Autodesk Inventor part; units mm, degrees
ref_plane "YZ Plane" through (0, 0, 0) normal (1, 0, 0) x (0, 1, 0)
ref_plane "XZ Plane" through (0, 0, 0) normal (0, 1, 0) x (-1, 0, 0)
ref_plane "XY Plane" through (0, 0, 0) normal (0, 0, 1) x (1, 0, 0)
sketch "Sketch1" plane through (0, 0, 0) normal (0, 0, 1) x (1, 0, 0)
  circle A0 centre (0, 0) radius 1.725
  dimension "d0" = 3.45
extrude "Extrusion1" add sketch "Sketch1" along normal blind 0.5
sketch "Sketch2" plane through (0, 0, 0.5) normal (0, 0, 1) x (1, 0, 0)
  circle A0 centre (0, 0) radius 1.725
  circle A1 centre (0, 0) radius 1.1
  dimension "d3" = 2.2
extrude "Extrusion2" add sketch "Sketch2" along normal blind 8 contours A1
fillet "Fillet1" radius 0.6 1 edges at (-1.1, 0, 8.5)
properties material "Copper"
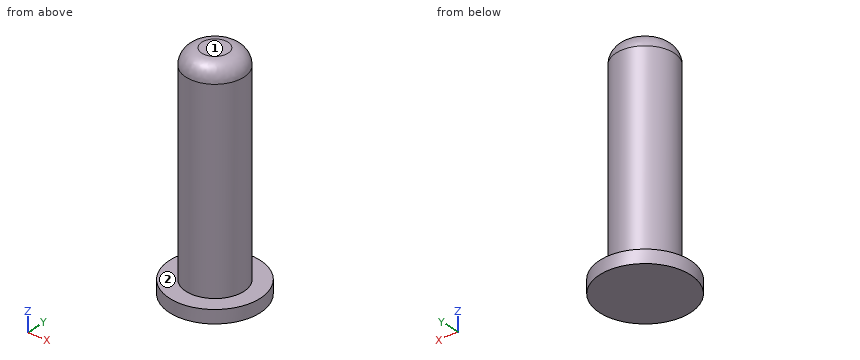
The model under review builds one solid part; all positions refer to its coordinate system, in mm. Face numbers are marked on the shaded views. A direction names the side the tool comes from. Round coordinates to 2 decimals unless told otherwise and drop trailing zeros. Loops run counter-clockwise (first coordinate to the right, second up) from the corner with the lowest first, then second, coordinate; pieces in that order, holes last. Notation, with made-up numbers: (-18.75, 26) -> (5.25, 26) arc R15 ccw to (5.25, 40) -> close; hole circle Ø4 at (27, -40). An arc over 180 degrees is marked (long way). Answer as a JSON object with one key per item and string values. Group by question number.
1) For the marked faces 1 and 2, list the 3-axis set-ups (+Z, -Z, +X, -X, +Y, -Y) from which the entire face can be reached by the end or side of a thin tool; tool diameter is ignored.
2) We need section A-A on z = 4.25. Write out the cut boundary in (x, y).
3) We need section C-C on y = -1.35. Write out the cut boundary in (x, z).
4) We need section B-B on x = 1.2. Write out the cut boundary in (y, z).
5) For line 1 (Z direction, x = -1.4, y = 0.7); line 2 (X direction, y = -0.05, z = 5.25); line 3 (Y direction, x = -0.55, z = 5), list the stretches that pass through material, from the lowest coordinate up. Write a range as [from, to].
Result set:
{
 "1": {"face 1": "+Z, +X, -X, +Y, -Y", "face 2": "+Z"},
 "2": {"outline": "circle Ø2.2 at (0, 0)"},
 "3": {"outline": "(-1.07, 0) -> (1.07, 0) -> (1.07, 0.5) -> (-1.07, 0.5) -> close"},
 "4": {"outline": "(-1.24, 0) -> (1.24, 0) -> (1.24, 0.5) -> (-1.24, 0.5) -> close"},
 "5": {"line 1": "[0, 0.5]", "line 2": "[-1.1, 1.1]", "line 3": "[-0.95, 0.95]"}
}
